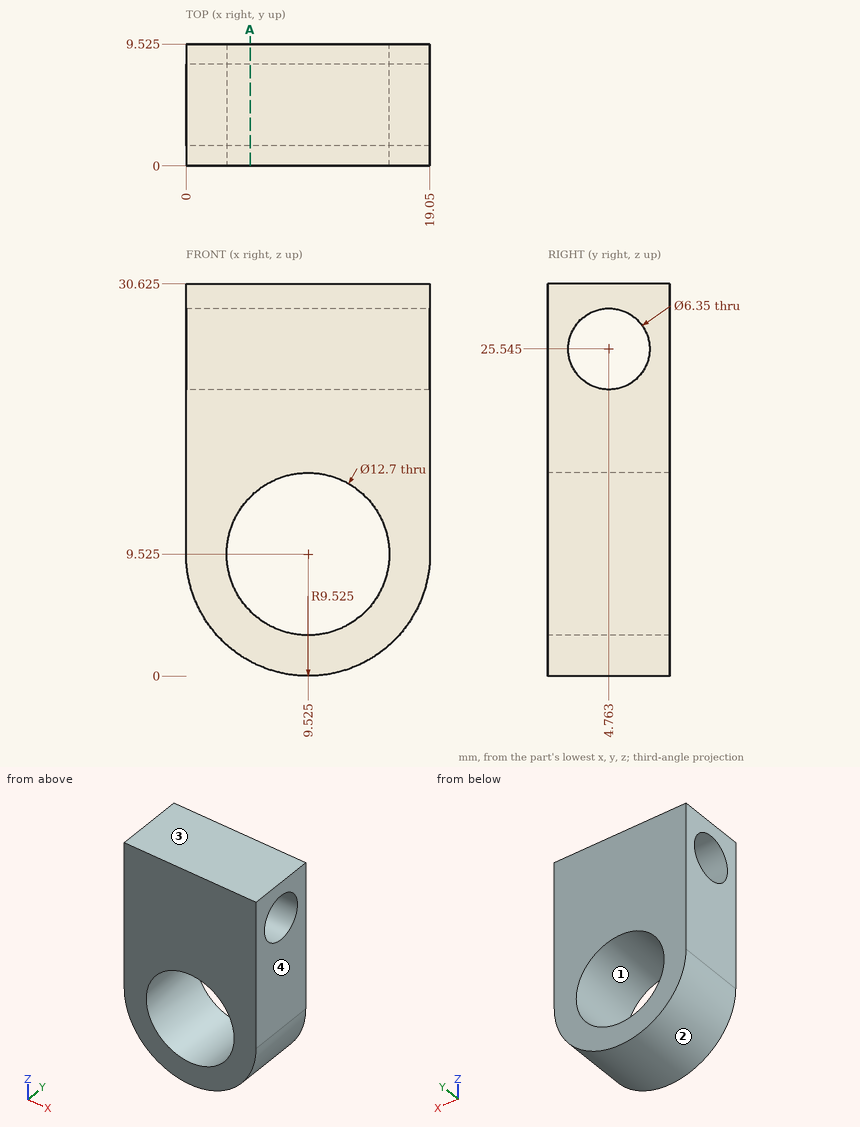
The drawing under review shows one solid part. Ordinate dimensions are in mm from its lowest x, y, z. Coordinates: 2 decimals unless noted, no trailing zeros. Use one line per item in the form item = value.
Q1. Insertion check: pin 1 Ø1 at (y, z) = (7, 7.5) entering from -X; pin 2 Ø2 at (y, z) = (7.5, 3.5) entering from -X. Each pin has a flat end and moves straight along its axis. Give the tip position at first contact, or say it passes through.
Taken from the geometry:
pin_1 = 0.12
pin_2 = 1.43
Q2. Consider section A-A (x = 5). Count the separate pieces of the cut face and the enclosed holes in it, plus the area to 3 significant figures.
Taken from the geometry:
separate_pieces = 2
enclosed_holes = 1
area = 164 mm^2
Q3. For probe 1 along Z at (x, y) = (4.75, 3.5) (1 decimal); probe 2 along Y at (x, z) = (3.75, 25.5) (1 decimal); probe 3 along Y at (x, z) = (11.75, 27.5) (1 decimal), list the stretches that pass through material, from the lowest coordinate up.
Taken from the geometry:
probe_1 = 1.3 to 5.3, 13.7 to 22.6, 28.5 to 30.6
probe_2 = 0 to 1.6, 7.9 to 9.5
probe_3 = 0 to 2.3, 7.3 to 9.5
Q4. The part is to be moulded in two halves that separate along X. For the marked faces 1, 2, 3 and 4, say which applies: +X half, -X half, draft (parallel to the pull), parting line (faces both ways), or undercut.
Taken from the geometry:
face_1 = undercut
face_2 = parting line
face_3 = draft
face_4 = +X half
